Autodesk Inventor part; units mm, degrees
ref_plane "YZ Plane" through (0, 0, 0) normal (1, 0, 0) x (0, 1, 0)
ref_plane "XZ Plane" through (0, 0, 0) normal (0, 1, 0) x (-1, 0, 0)
ref_plane "XY Plane" through (0, 0, 0) normal (0, 0, 1) x (1, 0, 0)
sketch "Sketch1" plane through (0, 0, 0) normal (0, 0, 1) x (1, 0, 0)
  line L0 (0, 0) -> (50, 0)
  line L1 (50, 0) -> (50, -25)
  line L2 (50, -25) -> (0, -25)
  line L3 (0, -25) -> (0, 0)
  dimension "d0" = 50
  dimension "d1" = 25
extrude "Extrusion1" add sketch "Sketch1" along normal blind 2
sketch "Sketch2" plane through (0, 0, 2) normal (0, 0, 1) x (1, 0, 0)
  line L0 (47.85, -2.15) -> (2.15, -2.15)
  line L1 (2.15, -2.15) -> (2.15, -22.85)
  line L2 (2.15, -22.85) -> (47.85, -22.85)
  line L3 (47.85, -22.85) -> (47.85, -2.15)
  line L4 (50, -25) -> (50, 0)
  line L5 (50, 0) -> (0, 0)
  dimension "d4" = 45.7
  dimension "d5" = 20.7
  dimension "d6" = 2.15
  dimension "d7" = 2.15
extrude "Extrusion2" add sketch "Sketch2" along normal blind 2
sketch "Sketch3" plane through (0, 0, 0) normal (0, 0, -1) x (-1, 0, 0)
  line L0 (0, -25) -> (-50, -25)
  line L1 (-19, -25) -> (-31, -25)
  line L2 (-31, -25) -> (-31, -17)
  line L3 (-31, -17) -> (-19, -17)
  line L4 (-19, -17) -> (-19, -25)
  line L5 (0, 0) -> (0, -25)
  dimension "d10" = 12
  dimension "d11" = 8
  dimension "d12" = 19
extrude "Extrusion3" cut sketch "Sketch3" against normal through all
chamfer "Chamfer1" distance 0.5 angle 45 5 edges at (25, -2.15, 4) (47.85, -12.5, 4) (39.425, -22.85, 4) (10.575, -22.85, 4) (2.15, -12.5, 4)
properties part number "UltrasonicSensorMountTest_backplate"
Can you work these out from the model? Positions are in its coordinate system, mm. A direction names the side the tool comes from. Round coordinates to 2 decimals unless told otherwise and drop trailing zeros. Order: outer loops, then holes, each group sorted by start corner. A loop starts at its lowest first (then second) coordinate and runs counter-clockwise, first axis right, second up. Notation, with made-up numbers: (48.25, 82.5) -> (89.25, 82.5) arc R26 ccw to (89.25, 112.5) -> close; hole circle Ø10 at (-16.75, -19). An arc over 180 degrees is marked (long way). Return JSON: item names as keys, results as strings. Group by question number.
1. Will these pins go through, and if not, where does the flat tip stop? pin 1 (1 mm diameter, centred on x = 11.5, z = 0.5, fed in from +Y); pin 2 (0.8 mm diameter, centred on y = -15.5, z = 3, fed in from -X); pin 3 (2 mm diameter, centred on x = 23, z = 3, fed in from -Y); pin 4 (0.8 mm diameter, centred on y = -8, z = 3, fed in from +X).
2. If we section it at A-A, the plane y = -20: Write out the boundary of the cut face in (x, z), then the cut area to 3 significant figures.
3. Which directions (+Z, -Z, +X, -X, +Y, -Y) give clear straight access to the entire face, cutting with the end or side of a thin tool? Please do faces 4 (the face through (25, -2.15, 3)), 5 (the face through (10, -22.85, 3)), 6 (the face through (25, -17, 2)).
4. If we section it at D-D, the plane y = -10.75: Write out the boundary of the cut face in (x, z), then the cut area to 3 significant figures.
5. I need wall thicknesses on line 1 (X direction, y = -18.25, z = 0.9); line 2 (X direction, y = -19.5, z = 2.75); line 3 (X direction, y = -13.75, z = 2.4). Which ranges of each line are inside material? Lowest first, please. Write a range as [from, to].
6. If we section it at C-C, the plane z = 2.9: Write out the boundary of the cut face in (x, y), then the cut area to 3 significant figures.
7. If we section it at B-B, the plane x = 30: Write out the boundary of the cut face in (y, z).
8. We'd pull the mould along X, two halves only. Please class faces 1 (the face through (31, -21, 2)), 2 (the face through (47.85, -13, 3)), 3 (the face through (23, -1, 2)): released by +X, released by -X, zero draft, split by the parting line, or undercut.
Output values:
{
 "1": {"pin 1": "y = 0", "pin 2": "x = 2.15", "pin 3": "y = -17", "pin 4": "x = 47.85"},
 "2": {"outline": "(0, 0) -> (19, 0) -> (19, 4) -> (2.65, 4) -> (2.15, 3.5) -> (2.15, 2) -> (0, 2) -> close; (31, 0) -> (50, 0) -> (50, 2) -> (47.85, 2) -> (47.85, 3.5) -> (47.35, 4) -> (31, 4) -> close", "area": "143 mm²"},
 "3": {"face 4": "+Z, +X, -X, +Y", "face 5": "+Z, +X, -X, -Y", "face 6": "+Z, -Z, -Y"},
 "4": {"outline": "(0, 0) -> (50, 0) -> (50, 2) -> (47.85, 2) -> (47.85, 3.5) -> (47.35, 4) -> (2.65, 4) -> (2.15, 3.5) -> (2.15, 2) -> (0, 2) -> close", "area": "191 mm²"},
 "5": {"line 1": "[0, 19], [31, 50]", "line 2": "[2.15, 19], [31, 47.85]", "line 3": "[2.15, 47.85]"},
 "6": {"outline": "(2.15, -22.85) -> (19, -22.85) -> (19, -17) -> (31, -17) -> (31, -22.85) -> (47.85, -22.85) -> (47.85, -2.15) -> (2.15, -2.15) -> close", "area": "876 mm²"},
 "7": {"outline": "(-17, 0) -> (0, 0) -> (0, 2) -> (-2.15, 2) -> (-2.15, 3.5) -> (-2.65, 4) -> (-17, 4) -> close"},
 "8": {"face 1": "undercut", "face 2": "released by +X", "face 3": "zero draft"}
}
